Can you work these out from the model? Positions are in its coordinate system, mm. A direction names the side the tool comes from. Round coordinates to 2 decimals unless told otherwise and drop trailing zeros. Order: outer loops, then holes, each group sorted by start corner. A loop starts at its lowest first (then second) coordinate and runs counter-clockwise, first axis right, second up. Notation, with made-up numbers: (-37.5, 18.25) - (-27.5, 18.25) arc R15 ccw to (-27.5, 31.25) - close; hole circle Ø11 at (12.5, 56.5). An arc over 180 degrees is marked (long way). Write item = value, one per line.
from build123d import *

# Parameters (mm, degrees)
BOSS_EXTRUDE1_DEPTH            = 48
CUT_EXTRUDE1_REACH             = 117.56
SKETCH5_R                      = 5
SKETCH5_R_2                    = 3
CUT_EXTRUDE1_DIRECTION_2_DEPTH = 116.559508479
SKETCH10_R                     = 12
SKETCH10_R_2                   = 2
CUT_EXTRUDE3_DEPTH             = 2
SKETCH15_W                     = 22
SKETCH15_H                     = 24
CUT_EXTRUDE5_DEPTH             = 2
BOSS_EXTRUDE7_DEPTH            = 93
BOSS_EXTRUDE7_DEPTH_BACK       = 2
SKETCH16_W                     = 24
SKETCH16_H                     = 2
FILLET1_R                      = 10


with BuildPart() as part:
    # Sketch1 → Boss-Extrude1 (new body)
    with BuildSketch(Plane.XY):
        Polygon((-1, 2.5), (-1, -45.5), (-45, -45.5), (-45, -47.5), (-1, -47.5), (1, -47.5), (0.957894737, -45.5), (1, -45.5), (1, 2.5), (1, 4.5), (1, 45.5), (1, 47.5), (-1, 47.5), (-45, 47.5), (-45, 45.5), (-1, 45.5), (-1, 4.5), (-45, 4.5), (-45, 2.5), align=None)
    extrude(amount=-BOSS_EXTRUDE1_DEPTH)

    # Sketch5 → Cut-Extrude1 (cut, up to next)
    with BuildSketch(Plane(origin=(0, 47.5, 0), x_dir=(1, 0, 0), z_dir=(0, 1, 0)), mode=Mode.PRIVATE) as cut_extrude1_sk1:
        with Locations(Location((-23, 24, 0), (0, 0, 90))):
            Circle(SKETCH5_R)
    cut_extrude1_tool1 = extrude(cut_extrude1_sk1.sketch, amount=-CUT_EXTRUDE1_REACH, mode=Mode.PRIVATE) & part.part
    # Sketch5 → Cut-Extrude1 (cut, up to next)
    with BuildSketch(Plane(origin=(0, 47.5, 0), x_dir=(1, 0, 0), z_dir=(0, 1, 0)), mode=Mode.PRIVATE) as cut_extrude1_sk2:
        with Locations(Location((-38.5, 39.5, 0), (0, 0, 90))):
            Circle(SKETCH5_R_2)
    cut_extrude1_tool2 = extrude(cut_extrude1_sk2.sketch, amount=-CUT_EXTRUDE1_REACH, mode=Mode.PRIVATE) & part.part
    # Sketch5 → Cut-Extrude1 (cut, up to next)
    with BuildSketch(Plane(origin=(0, 47.5, 0), x_dir=(1, 0, 0), z_dir=(0, 1, 0)), mode=Mode.PRIVATE) as cut_extrude1_sk3:
        with Locations(Location((-7.5, 39.5, 0), (0, 0, 90))):
            Circle(SKETCH5_R_2)
    cut_extrude1_tool3 = extrude(cut_extrude1_sk3.sketch, amount=-CUT_EXTRUDE1_REACH, mode=Mode.PRIVATE) & part.part
    # Sketch5 → Cut-Extrude1 (cut, up to next)
    with BuildSketch(Plane(origin=(0, 47.5, 0), x_dir=(1, 0, 0), z_dir=(0, 1, 0)), mode=Mode.PRIVATE) as cut_extrude1_sk4:
        with Locations(Location((-7.5, 8.5, 0), (0, 0, 90))):
            Circle(SKETCH5_R_2)
    cut_extrude1_tool4 = extrude(cut_extrude1_sk4.sketch, amount=-CUT_EXTRUDE1_REACH, mode=Mode.PRIVATE) & part.part
    # Sketch5 → Cut-Extrude1 (cut, up to next)
    with BuildSketch(Plane(origin=(0, 47.5, 0), x_dir=(1, 0, 0), z_dir=(0, 1, 0)), mode=Mode.PRIVATE) as cut_extrude1_sk5:
        with Locations(Location((-38.5, 8.5, 0), (0, 0, 90))):
            Circle(SKETCH5_R_2)
    cut_extrude1_tool5 = extrude(cut_extrude1_sk5.sketch, amount=-CUT_EXTRUDE1_REACH, mode=Mode.PRIVATE) & part.part
    add(cut_extrude1_tool1.solids().sort_by_distance((-23, 47.5, -24))[0], mode=Mode.SUBTRACT)
    add(cut_extrude1_tool2.solids().sort_by_distance((-38.5, 47.5, -39.5))[0], mode=Mode.SUBTRACT)
    add(cut_extrude1_tool3.solids().sort_by_distance((-7.5, 47.5, -39.5))[0], mode=Mode.SUBTRACT)
    add(cut_extrude1_tool4.solids().sort_by_distance((-7.5, 47.5, -8.5))[0], mode=Mode.SUBTRACT)
    add(cut_extrude1_tool5.solids().sort_by_distance((-38.5, 47.5, -8.5))[0], mode=Mode.SUBTRACT)

    # Sketch5 → Cut-Extrude1 direction 2 (cut)
    with BuildSketch(Plane(origin=(0, 47.5, 0), x_dir=(1, 0, 0), z_dir=(0, 1, 0))):
        with Locations(Location((-23, 24, 0), (0, 0, 90))):
            Circle(SKETCH5_R)
        with Locations(Location((-38.5, 39.5, 0), (0, 0, 90))):
            Circle(SKETCH5_R_2)
        with Locations(Location((-7.5, 39.5, 0), (0, 0, 90))):
            Circle(SKETCH5_R_2)
        with Locations(Location((-7.5, 8.5, 0), (0, 0, 90))):
            Circle(SKETCH5_R_2)
        with Locations(Location((-38.5, 8.5, 0), (0, 0, 90))):
            Circle(SKETCH5_R_2)
    extrude(amount=CUT_EXTRUDE1_DIRECTION_2_DEPTH, mode=Mode.SUBTRACT)

    # Sketch10 → Cut-Extrude3 (cut)
    with BuildSketch(Plane(origin=(0, 4.5, 0), x_dir=(1, 0, 0), z_dir=(0, 1, 0))):
        with Locations(Location((-23, 24, 0), (0, 0, 180))):
            Circle(SKETCH10_R)
        with Locations(Location((-7.5, 39.5, 0), (0, 0, 180))):
            Circle(SKETCH10_R_2)
        with Locations(Location((-7.5, 8.5, 0), (0, 0, 180))):
            Circle(SKETCH10_R_2)
        with Locations(Location((-38.5, 8.5, 0), (0, 0, 180))):
            Circle(SKETCH10_R_2)
        with Locations(Location((-38.5, 39.5, 0), (0, 0, 180))):
            Circle(SKETCH10_R_2)
    extrude(amount=-CUT_EXTRUDE3_DEPTH, mode=Mode.SUBTRACT)

    # Sketch15 → Cut-Extrude5 (cut)
    with BuildSketch(Plane(origin=(0, 4.5, 0), x_dir=(1, 0, 0), z_dir=(0, 1, 0))):
        with Locations((-34, 24)):
            Rectangle(SKETCH15_W, SKETCH15_H)
    extrude(amount=-CUT_EXTRUDE5_DEPTH, mode=Mode.SUBTRACT)

    # Sketch16 → Boss-Extrude7 (add, two sides: drawn at the far end of the back side and taken through both)
    with BuildSketch(Plane(origin=(0, -45.5, 0), x_dir=(1, 0, 0), z_dir=(0, 1, 0)).offset(-BOSS_EXTRUDE7_DEPTH_BACK)):
        with Locations((-11, 1)):
            Rectangle(SKETCH16_W, SKETCH16_H)
        with Locations((-11, 47)):
            Rectangle(SKETCH16_W, SKETCH16_H)
    extrude(amount=BOSS_EXTRUDE7_DEPTH + BOSS_EXTRUDE7_DEPTH_BACK)

    # Fillet1
    fillet1_edges = [part.edges().sort_by_distance(p)[0] for p in [
        (-23, -45.5, -1),
        (-23, 2.5, -1),
        (-23, 4.5, -1),
        (-23, 45.5, -1),
        (-23, -45.5, -47),
        (-23, 2.5, -47),
        (-23, 4.5, -47),
        (-23, 45.5, -47),
    ]]
    fillet(fillet1_edges, radius=FILLET1_R)


solid = part.part
(1) On a 3-axis mill with a long thin cutter (end or side, diameter ignored), from which of +Z, -Z, +X, -X, +Y, -Y can I reach the whole of each face in a straight line? I mean faces 4 (the face through (-23, -45.5, -24)), 5 (the face through (-45, 47, -24)), 6 (the face through (-25.85, 42.49, -47.01)), 7 (the face through (-37.026, 3.514, -7.148)). Say none if no direction works.
Computed:
face_4 = -X
face_5 = +Z, -Z, -X, +Y, -Y
face_6 = +Z, -Z, -X
face_7 = +Y
(2) If I drill on line 1 (Y direction, x = -6, z = -19.5); line 2 (X direction, y = 47, z = -8.5); line 3 (Z direction, x = -38.5, y = 3.95), over which ranges is the centre line in solid material (lowest first)? Write a range as from..to.
Computed:
line_1 = -47.5..-45.5, 2.5..4.5, 45.5..47.5
line_2 = -45..-41.5, -35.5..-10.5, -4.5..1
line_3 = -48..-41.5, -37.5..-36, -12..-10.5, -6.5..0
(3) If we section it at D-D (x = -3): Write out the boundary of the cut face in (y, z).
Computed:
outline = (-47.5, -48) - (47.5, -48) - (47.5, 0) - (-47.5, 0) - close; hole (-45.5, -46) - (2.5, -46) - (2.5, -2) - (-45.5, -2) - close; hole (4.5, -46) - (45.5, -46) - (45.5, -2) - (4.5, -2) - close
(4) If we section it at A-A (z = -24): Write out the boundary of the cut face in (x, y), plus the area to 3 significant figures.
Computed:
outline = (-45, -47.5) - (1, -47.5) - (0.96, -45.5) - (1, -45.5) - (1, 47.5) - (-18, 47.5) - (-18, 45.5) - (-1, 45.5) - (-1, 4.5) - (-11, 4.5) - (-11, 2.5) - (-1, 2.5) - (-1, -45.5) - (-45, -45.5) - close; (-45, 45.5) - (-28, 45.5) - (-28, 47.5) - (-45, 47.5) - close
area = 366 mm^2
(5) If we section it at C-C (z = -8.5): State how many separate pieces and enclosed holes the cut face has, plus the area to 3 significant figures.
Computed:
separate_pieces = 5
enclosed_holes = 0
area = 414 mm^2
(6) Thinking about a two-plate mould opening in Z: for faces 1 (the face through (-12, 1, -48)), 2 (the face through (-25.85, 42.49, -1.01)), 3 (the face through (-9, 2.5, -24)), which applies, +Z half, -Z half, draft (parallel to the pull), parting line (faces both ways), or undercut?
Computed:
face_1 = -Z half
face_2 = draft
face_3 = undercut
(7) If we section it at B-B (x = -34): Write out the boundary of the cut face in (y, z).
Computed:
outline = (-47.5, -48) - (-45.5, -48) - (-45.5, 0) - (-47.5, 0) - close; (2.5, -48) - (4.5, -48) - (4.5, -36) - (2.5, -36) - close; (2.5, -12) - (4.5, -12) - (4.5, 0) - (2.5, 0) - close; (45.5, -48) - (47.5, -48) - (47.5, 0) - (45.5, 0) - close
(8) Will these pins go through, and if not, where does the flat tip stop? P1, Ø3.5, axis at x = -7.5, z = -8.5, coming from the +Y side; P2, Ø5, axis at x = -38.5, z = -8.5, coming from the +Y side; P3, Ø5, axis at y = -37.5, z = -38, coming from the -X side; P4, Ø2, axis at x = -31.5, y = 3, coming from the +Z side.
Computed:
P1 = -45.5
P2 = 4.5
P3 = -1
P4 = 0
